Could you check a few things on this model? Use its own coordinates, in mm. A direction names the side the tool comes from. Coordinates: 2 decimals unless noted, no trailing zeros. Loops run counter-clockwise (first coordinate to the right, second up) from the corner with the lowest first, then second, coordinate; pieces in that order, holes last. Notation, with made-up numbers: (52, 18.25) - (66, 18.25) arc R18 cw to (66, 26.25) - close; hole circle Ø3 at (25.25, 75.25). An arc over 180 degrees is marked (long way). One line per item, written item: value. Start each with the question number.
(1) If we section it at C-C on z = 4.05: Write out the boundary of the cut face in (x, y).
(2) If I drill on line 1 along Y through (x, z) = (-15.5, 2.2); line 2 along Y through (x, z) = (-20, 0.85); line 3 along X through (y, z) = (48, 4.3), over which ranges is the centre line in solid material (lowest first)? Write a range as from..to.
(3) I'm going to push flat-ended pins straight in: P1, Ø1, axis at x = -14, z = 1, coming from the -Y side; P2, Ø3, axis at x = -17.5, z = 1.5, coming from the -Y side; P3, Ø2.5, axis at x = -15.5, y = -15.5, coming from the -Z side; P4, Ø1, axis at x = -21.5, z = 3.5, coming from the +Y side. Where does each tip first touch, or does it pass through?
(4) If we section it at A-A on x = -15.5: Write out the boundary of the cut face in (y, z), then the cut area to 4 significant figures.
(5) If we section it at B-B on y = 0: Write out the boundary of the cut face in (x, z), then the cut area to 3 significant figures.
(6) On a 3-axis mill with a long thin cutter (end or side, diameter ignored), from which of +Z, -Z, +X, -X, +Y, -Y can I reach the whole of each face in a straight line? I mean faces 4 (the face through (-22, 41, 3)), 5 (the face through (-8.5, 15, 2)). Say none if no direction works.
(7) If we mould it in two halves opening along Y, with no side actions, what happens to faces 1 (the face through (-22, 38, 3)), 2 (the face through (-22.5, 43, 2)), 3 (the face through (-15.65, 51.5, 2.46))? For each: pulls with the +Y half, pulls with the -Y half, needs draft (parallel to the pull), parting line crosses it, or undercut.
```python
from build123d import *

# Parameters (mm, degrees)
BOSS_EXTRUDE1_DEPTH = 5
SKETCH2_R           = 1
CUT_EXTRUDE1_DEPTH  = 5
SKETCH3_W           = 3
SKETCH3_H           = 3
CUT_EXTRUDE2_DEPTH  = 5
FILLET1_R           = 1
SKETCH4_R           = 1.45
CUT_EXTRUDE3_DEPTH  = 5


with BuildPart() as part:
    # Sketch1 → Boss-Extrude1 (new body)
    with BuildSketch(Plane.XY):
        with BuildLine():
            Line((-22.5, -15.5), (-22.5, 44.5))
            ThreePointArc((-22.5, 44.5), (-15.5, 51.5), (-8.5, 44.5))
            Line((-8.5, 44.5), (-8.5, -15.5))
            ThreePointArc((-8.5, -15.5), (-15.5, -22.5), (-22.5, -15.5))
        make_face()
    extrude(amount=BOSS_EXTRUDE1_DEPTH)

    # Sketch2 → Cut-Extrude1 (cut)
    with BuildSketch(Plane.XY.offset(5)):
        with Locations((-12.75, 0)):
            Circle(SKETCH2_R)
    extrude(amount=-CUT_EXTRUDE1_DEPTH, mode=Mode.SUBTRACT)

    # Sketch3 → Cut-Extrude2 (cut)
    with BuildSketch(Plane.XY.offset(5)):
        with Locations((-21, 39.5)):
            Rectangle(SKETCH3_W, SKETCH3_H)
    extrude(amount=-CUT_EXTRUDE2_DEPTH, mode=Mode.SUBTRACT)

    # Fillet1
    fillet1_edges = [part.edges().sort_by_distance(p)[0] for p in [
        (-19.5, 41, 2.5),
        (-19.5, 38, 2.5),
    ]]
    fillet(fillet1_edges, radius=FILLET1_R)

    # Sketch4 → Cut-Extrude3 (cut)
    with BuildSketch(Plane.XY.offset(5)):
        with Locations((-15.5, -15.5)):
            Circle(SKETCH4_R)
    extrude(amount=-CUT_EXTRUDE3_DEPTH, mode=Mode.SUBTRACT)


solid = part.part
```
Values:
1. outline: (-22.5, -15.5) arc R7 ccw to (-8.5, -15.5) - (-8.5, 44.5) arc R7 ccw to (-22.5, 44.5) - (-22.5, 41) - (-20.5, 41) arc R1 cw to (-19.5, 40) - (-19.5, 39) arc R1 cw to (-20.5, 38) - (-22.5, 38) - close; hole circle Ø2.9 at (-15.5, -15.5); hole circle Ø2 at (-12.75, 0)
2. line 1: y = -22.5..-16.95, -14.05..51.5
2. line 2: y = -20.86..38.13, 40.87..49.86
2. line 3: x = -21.56..-9.44
3. P1: stops at y = -22.43
3. P2: stops at y = -22.48
3. P3: passes through
3. P4: stops at y = 48.83
4. outline: (-22.5, 0) - (-16.95, 0) - (-16.95, 5) - (-22.5, 5) - close; (-14.05, 0) - (51.5, 0) - (51.5, 5) - (-14.05, 5) - close
4. area: 355.5 mm2
5. outline: (-22.5, 0) - (-13.75, 0) - (-13.75, 5) - (-22.5, 5) - close; (-11.75, 0) - (-8.5, 0) - (-8.5, 5) - (-11.75, 5) - close
5. area: 60.0 mm2
6. face 4: +Z, -Z, -X
6. face 5: +Z, -Z, +X, +Y, -Y
7. face 1: undercut
7. face 2: needs draft
7. face 3: pulls with the +Y half
